Read the model definition and answer for the solid it produces. Units are mm, in the model's axes. Face numbers are marked on the shaded views. Give positions to 0.01 mm unless a question says otherwise; leave off trailing zeros. Write each loop counter-clockwise with the first axis right and the second up, starting at its lowest first coordinate (ties: lowest second). Pieces come first, ordered by that corner, then holes. Notation, with made-up numbers: M 7.25,-6 L 15.25,-6 A25 ccw 15.25,18 Z; hole C 41,-36 d10. An arc over 180 degrees is marked long. Use a Markdown table: item, result. Add a question column.
Item 1: A cutting plane is placed at A-A on x = 53.75. Determine the outline of the cut face in (y, z), then the cut area to 3 significant figures.
Item 2: The mould has two halves that part along Y. Classify the marked faces 1, 2, 3 and 4: pulls with the +Y half, pulls with the -Y half, needs draft (parallel to the pull), parting line crosses it, or undercut.
Item 3: Given P1, Ø0.6, axis at y = 0.5, z = 149.5, coming from the +X side, flat-ended and moving along its own axis, determine where the tip first touches the part or whether it passes through.
Item 4: Consider probe 1 along Y at (x, z) = (54.75, 149.5); probe 2 along Z at (x, y) = (52, 1.5). Determine where each line is inside the solid, lowest interval first. Write a range as [from, to].
Item 5: A cutting plane is placed at B-B on y = 0. Determine the outline of the cut face in (x, z).
Item 6: A cutting plane is placed at C-C on z = 150.25. Determine the outline of the cut face in (x, y), then the cut area to 3 significant figures.
Item 7: A cutting plane is placed at D-D on x = 52.25. Determine the outline of the cut face in (y, z), then the cut area to 3 significant figures.
from build123d import *

# Parameters (mm, degrees)
BOSS_EXTRUDE1_START = 144
SKETCH1_W           = 6.2
SKETCH1_H           = 12
BOSS_EXTRUDE1_DEPTH = 12
BOSS_EXTRUDE2_START = 149
SKETCH2_W           = 2.8
SKETCH2_H           = 3.9
BOSS_EXTRUDE2_DEPTH = 1.6
BOSS_EXTRUDE3_START = 149
SKETCH3_W           = 1.7
SKETCH3_H           = 3.9
BOSS_EXTRUDE3_DEPTH = 2.1


with BuildPart() as part:
    # Sketch1 → Boss-Extrude1 (new body)
    with BuildSketch(Plane.XY.offset(BOSS_EXTRUDE1_START)):
        with Locations((52.5, 0)):
            Rectangle(SKETCH1_W, SKETCH1_H)
    extrude(amount=BOSS_EXTRUDE1_DEPTH)


with BuildPart() as body_2:
    # Sketch2 → Boss-Extrude2 (new body)
    with BuildSketch(Plane.XY.offset(BOSS_EXTRUDE2_START)):
        with Locations((54.3, 0)):
            Rectangle(SKETCH2_W, SKETCH2_H)
    extrude(amount=BOSS_EXTRUDE2_DEPTH)


with BuildPart() as part_1:
    add(part.part)

    # Combine1: cut body 2
    add(body_2.part, mode=Mode.SUBTRACT)


with BuildPart() as body_2_2:
    # Sketch3 → Boss-Extrude3 (new body)
    with BuildSketch(Plane.XY.offset(BOSS_EXTRUDE3_START)):
        with Locations((52.05, 0)):
            Rectangle(SKETCH3_W, SKETCH3_H)
    extrude(amount=BOSS_EXTRUDE3_DEPTH)


with BuildPart() as part_2:
    add(part_1.part)

    # Combine2: cut body 2 2
    add(body_2_2.part, mode=Mode.SUBTRACT)


solid = part_2.part
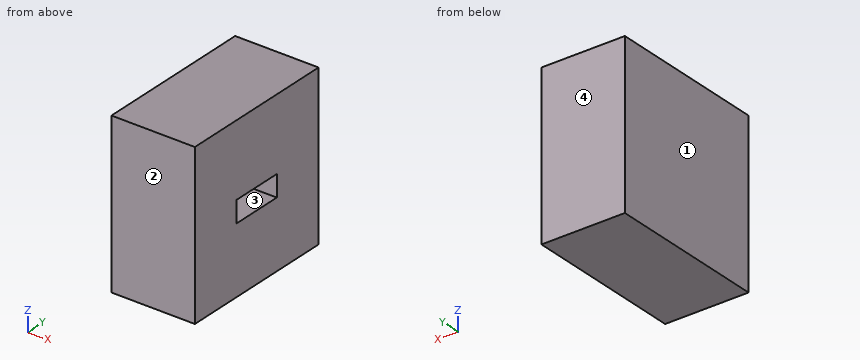
Filled in:
| question | item | result |
|---|---|---|
| 1 | outline | M -6,144 L 6,144 L 6,156 L -6,156 Z; hole M -1.95,149 L 1.95,149 L 1.95,150.6 L -1.95,150.6 Z |
| 1 | area | 138 mm² |
| 2 | face 1 | needs draft |
| 2 | face 2 | pulls with the -Y half |
| 2 | face 3 | undercut |
| 2 | face 4 | pulls with the +Y half |
| 3 | P1 | x = 51.2 |
| 4 | probe 1 | [-6, -1.95], [1.95, 6] |
| 4 | probe 2 | [144, 149], [151.1, 156] |
| 5 | outline | M 49.4,144 L 55.6,144 L 55.6,149 L 51.2,149 L 51.2,151.1 L 52.9,151.1 L 52.9,150.6 L 55.6,150.6 L 55.6,156 L 49.4,156 Z |
| 6 | outline | M 49.4,-6 L 55.6,-6 L 55.6,-1.95 L 51.2,-1.95 L 51.2,1.95 L 55.6,1.95 L 55.6,6 L 49.4,6 Z |
| 6 | area | 57.2 mm² |
| 7 | outline | M -6,144 L 6,144 L 6,156 L -6,156 Z; hole M -1.95,149 L 1.95,149 L 1.95,151.1 L -1.95,151.1 Z |
| 7 | area | 136 mm² |
